Model file for the job. Use its own axes, mm. A direction names the side the tool comes from. Give positions to 0.01 mm unless a question says otherwise; leave off trailing zeros. Order: outer loops, then holes, each group sorted by start corner. A loop starts at its lowest first (then second) coordinate and runs counter-clockwise, first axis right, second up. Notation, with made-up numbers: (16.5, -3) - (44.5, -3) arc R19 cw to (44.5, 24) - close; hole circle Ø11 at (5, 78). An arc over 180 degrees is marked (long way). Use CSV: the item, a comma, the result in double quotes. Start each with the question number.
(1) Band-saw the part on A-A, the plane y = 126.5. Give the cut face in (x, z), then the cut area to 3 significant figures.
(2) Band-saw the part on B-B, the plane x = -248. Give the cut face in (y, z), then the cut area to 3 significant figures.
(3) Band-saw the part on C-C, the plane z = -297. Give the cut face in (x, y).
(4) Pull direction X, two halves, no side cores. Call faces 1 (the flat face through (-155, 12.7, -309)), 2 (the flat face through (7, 139.7, -209)), 3 (the flat face through (-317.5, 69, -309)): +X half, -X half, draft (parallel to the pull), parting line (faces both ways), or undercut.
(5) Tool access for faces 4 (the flat face through (-150, 0, -300)), 5 (the flat face through (0, 77, -309)): list every direction of +Z, -Z, +X, -X, +Y, -Y with a clear straight run to the whole face (end or side of a thin tool).
(6) Probe L1, parallel to X at y = 129, z = -353; L2, parallel to Z at x = -236, y = 19; L3, parallel to Y at x = -67.5, z = -332. List the from-to ranges inside material, lowest first.
Autodesk Inventor part; units mm, degrees
ref_plane "YZ Plane" through (0, 0, 0) normal (1, 0, 0) x (0, 1, 0)
ref_plane "XZ Plane" through (0, 0, 0) normal (0, 1, 0) x (-1, 0, 0)
ref_plane "XY Plane" through (0, 0, 0) normal (0, 0, 1) x (1, 0, 0)
sketch "Sketch1" plane through (0, 0, 0) normal (0, 1, 0) x (-1, 0, 0)
  line L0 (0, 0) -> (304.8, 0)
  line L1 (304.8, 0) -> (304.8, -609.6)
  line L2 (304.8, -609.6) -> (0, -609.6)
  line L3 (0, -609.6) -> (0, 0)
  line L4 (317.5, 12.7) -> (-12.7, 12.7)
  line L5 (-12.7, 12.7) -> (-12.7, -622.3)
  line L6 (-12.7, -622.3) -> (317.5, -622.3)
  line L7 (317.5, -622.3) -> (317.5, 12.7)
  dimension "d0" = 304.8
  dimension "d1" = 609.6
  dimension "d2" = 12.7
extrude "Extrusion1" add sketch "Sketch1" along normal blind 139.7 contours L0 L1 L2 L3 | L7 L6 L5 L4
sketch "Sketch2" plane through (0, 139.7, 0) normal (0, 1, 0) x (1, 0, 0)
  line L0 (0, 0) -> (-304.8, 0)
  line L1 (-304.8, 0) -> (-304.8, 609.6)
  line L2 (-304.8, 609.6) -> (0, 609.6)
  line L3 (0, 609.6) -> (0, 0)
  dimension "d5" = 304.8
  dimension "d6" = 609.6
extrude "Extrusion2" cut sketch "Sketch2" against normal blind 127
properties part number "PlantBox"
Answer block:
1,outline,"(-317.5, -622.3) - (12.7, -622.3) - (12.7, 12.7) - (-317.5, 12.7) - close; hole (-304.8, -609.6) - (0, -609.6) - (0, 0) - (-304.8, 0) - close"
1,area,"23,900 mm2"
2,outline,"(0, -622.3) - (139.7, -622.3) - (139.7, -609.6) - (12.7, -609.6) - (12.7, 0) - (139.7, 0) - (139.7, 12.7) - (0, 12.7) - close"
2,area,"11,300 mm2"
3,outline,"(-317.5, 0) - (12.7, 0) - (12.7, 139.7) - (0, 139.7) - (0, 12.7) - (-304.8, 12.7) - (-304.8, 139.7) - (-317.5, 139.7) - close"
4,face 1,"undercut"
4,face 2,"draft"
4,face 3,"-X half"
5,face 4,"+Z, -Z, +X, -X, -Y"
5,face 5,"+Y"
6,L1,"x = -317.5 to -304.8, 0 to 12.7"
6,L2,"z = -622.3 to -609.6, 0 to 12.7"
6,L3,"y = 0 to 12.7"
